```python
from build123d import *

# Parameters (mm, degrees)
F0_R     = 9
F1_DEPTH = 12
F2_SIZE2 = 4.5286636519
F2_SIZE  = 3.8
F3_R     = 0.6
F4_DEPTH = 9


with BuildPart() as f1:
    # F0 (on Front) → F1 (new body)
    with BuildSketch(Plane.XZ):
        Circle(F0_R)
    extrude(amount=F1_DEPTH)

    # F2
    f2_edges = [f1.edges().sort_by_distance(p)[0] for p in [
        (-9, 0, 0),
    ]]
    f2_side = f1.faces().sort_by_distance((0, 0, 0))[0]
    chamfer(f2_edges, length=F2_SIZE, length2=F2_SIZE2, reference=f2_side)

    # F3 (on face) → F4 (join)
    with BuildSketch(Plane.XZ.offset(12)):
        with Locations((-5, 0)):
            Circle(F3_R)
        with Locations((5, 0)):
            Circle(F3_R)
    extrude(amount=F4_DEPTH)


solid = f1.part
```
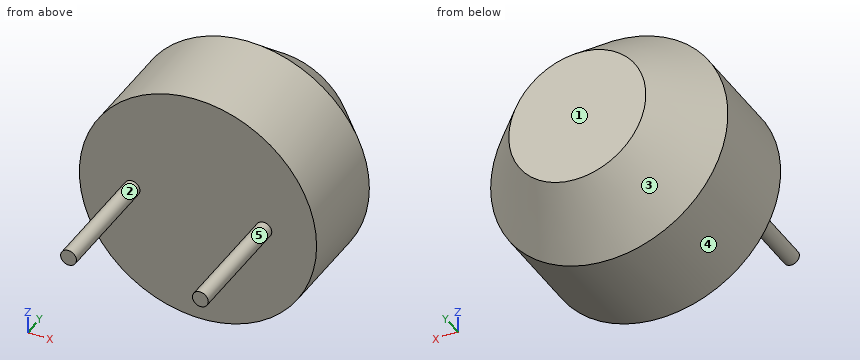
For this review, take the finished solid that the model builds, in its own axes (mm). Face numbers are marked on the shaded views. A direction names the side the tool comes from. Coordinates: 2 decimals unless noted, no trailing zeros. Loops run counter-clockwise (first coordinate to the right, second up) from the corner with the lowest first, then second, coordinate; pieces in that order, holes last.
1. Add section B-B, the plane z = 0. Give the boundary of the cut face in (x, y), then the cut area to 3 significant figures.
2. For the marked faces 4 and 5, list the 3-axis set-ups (+Z, -Z, +X, -X, +Y, -Y) from which the entire face can be reached by the end or side of a thin tool; tool diameter is ignored.
3. Insertion check: P1, Ø8, axis at x = 3.5, z = 7, coming from the -Y side; P2, Ø6, axis at y = -10.5, z = 7, coming from the -X side; P3, Ø2, axis at y = -7, z = -7, coming from the +X side; P4, Ø5, axis at x = -1.5, y = -17.5, coming from the -Z side. Each pin has a flat end and moves straight along its axis. Give the tip position at first contact, or say it passes through.
4. Mouldability with a two-part tool opening along X and no side actions: class the marked faces 1, 2 and 3 as +X half, -X half, draft (parallel to the pull), parting line (faces both ways), or undercut.
5. Add section D-D, the plane y = -6.5. Give the boundary of the cut face in (x, z), then the cut area to 3 significant figures.
6. Add section A-A, the plane y = -16.75. Give the boundary of the cut face in (x, z), then the cut area to 3 significant figures.
7. For line 1 (Y direction, x = 3, z = 2.5); line 2 (Z direction, x = 5, y = -16); line 3 (Z direction, x = -2.25, y = -9), list the stretches that pass through material, from the lowest coordinate up.
8. Add section C-C, the plane x = 0. Give the boundary of the cut face in (y, z), then the cut area to 3 significant figures.
Result:
1. outline: (-9, -12) - (-5.6, -12) - (-5.6, -21) - (-4.4, -21) - (-4.4, -12) - (4.4, -12) - (4.4, -21) - (5.6, -21) - (5.6, -12) - (9, -12) - (9, -4.53) - (5.2, 0) - (-5.2, 0) - (-9, -4.53) - close
1. area: 220 mm2
2. face 4: +Y, -Y
2. face 5: -Y
3. P1: stops at y = -12
3. P2: stops at x = -8.06
3. P3: stops at x = 6.71
3. P4: passes through
4. face 1: draft
4. face 2: undercut
4. face 3: parting line
5. outline: circle Ø18 at (0, 0)
5. area: 254 mm2
6. outline: circle Ø1.2 at (-5, 0); circle Ø1.2 at (5, 0)
6. area: 2.26 mm2
7. line 1: y = -12 to 0
7. line 2: z = -0.6 to 0.6
7. line 3: z = -8.71 to 8.71
8. outline: (-12, -9) - (-4.53, -9) - (0, -5.2) - (0, 5.2) - (-4.53, 9) - (-12, 9) - close
8. area: 199 mm2
